Input: part model. Units: mm. Frame: model coordinates. A direction names the side the tool comes from. Give positions to 0.01 mm unless a question says otherwise; leave off trailing zeros. Loops run counter-clockwise (first coordinate to the right, second up) from the corner with the lowest first, then second, coordinate; pieces in that order, holes last. Notation, with made-up numbers: M 6,-12.5 L 58,-12.5 A31 cw 58,26.5 Z; hole C -7,38.25 d9. An arc over 180 degrees is marked long. Answer as a JSON object with one key per item and string values. Group by question number.
1) Section query D-D on z = 8. Return loops of the section in (x, y), plus the area to 3 significant figures.
2) Draft query along Y for faces 1 (the cylindrical face through (-4.769, -21.477, 14.986)), 2 (the cylindrical face through (-19.57, -0.65, 14.99)), 3 (the flat face through (9, -9, 14)), 4 (the flat face through (2.2, -2.2, 12.1)). Return one class per face: +Y half, -Y half, draft (parallel to the pull), parting line (faces both ways), or undercut.
3) Section query A-A on y = 0. Return loops of the section in (x, z).
4) First-contact query: P1, Ø2, axis at x = 6.5, z = 12.5, coming from the -Y side; P2, Ø6, axis at x = 8, y = -10, coming from the -Z side; P3, Ø2, axis at y = 4, z = 8, coming from the +X side; P4, Ø9, axis at x = 0, y = 0, coming from the +Z side. Flat tips, straight axial feed; report the tip coordinate or a pass-through.
5) Access query for faces 5 (the cylindrical face through (-1.08, -4.88, 14.08)), 6 (the flat face through (-5.2, 0.3, 16)), 7 (the cylindrical face through (-2.38, -10.74, 6.66)). Directions: +Z, -Z, +X, -X, +Y, -Y. A direction counts if a zero-diameter tool reaches every point of the face in a straight line with its end or side. Return the directions, or none.
6) Ray query, L1, parallel to Y at x = 0, z = 15.3; L2, parallel to Z at x = -6.5, y = 14; L3, parallel to Y at x = -1, z = 9.25. Return the intervals inside material, ascending.
7) Section query C-C on x = 18. Return loops of the section in (y, z).
from build123d import *

# Parameters (mm, degrees)
SKETCH1_R                                            = 11
BOSS_EXTRUDE1_DEPTH                                  = 14
SKETCH2_R                                            = 22
BOSS_EXTRUDE2_DEPTH                                  = 2
M3_CLEARANCE_HOLE1_D                                 = 3.4
CBORE_FOR_M5_HEX_SOCKET_THIN_HEAD_CAP_SC_D           = 5.5
CBORE_FOR_M5_HEX_SOCKET_THIN_HEAD_CAP_SC_CBORE_D     = 10
CBORE_FOR_M5_HEX_SOCKET_THIN_HEAD_CAP_SC_CBORE_DEPTH = 3.9
FILLET1_R                                            = 0.5


with BuildPart() as part:
    # Sketch1 → Boss-Extrude1 (new body)
    with BuildSketch(Plane.XY):
        Circle(SKETCH1_R)
    extrude(amount=BOSS_EXTRUDE1_DEPTH)

    # Sketch2 → Boss-Extrude2 (add)
    with BuildSketch(Plane.XY.offset(14)):
        Circle(SKETCH2_R)
    extrude(amount=BOSS_EXTRUDE2_DEPTH)

    # M3 Clearance Hole1 (through all)
    with Locations(Plane.XY.offset(16)):
        with Locations((-18, 0), (0, 18), (18, 0), (0, -18)):
            Hole(M3_CLEARANCE_HOLE1_D / 2)

    # CBORE for M5 Hex Socket Thin Head Cap Screw1 (through all)
    with Locations(Plane.XY.offset(16)):
        with Locations((0, 0)):
            CounterBoreHole(CBORE_FOR_M5_HEX_SOCKET_THIN_HEAD_CAP_SC_D / 2, CBORE_FOR_M5_HEX_SOCKET_THIN_HEAD_CAP_SC_CBORE_D / 2, CBORE_FOR_M5_HEX_SOCKET_THIN_HEAD_CAP_SC_CBORE_DEPTH)

    # Fillet1
    fillet1_edges = [part.edges().sort_by_distance(p)[0] for p in [
        (-11, 0, 14),
    ]]
    fillet(fillet1_edges, radius=FILLET1_R)


solid = part.part
Output:
{
 "1": {"outline": "C 0,0 d22; hole C 0,0 d5.5", "area": "356 mm^2"},
 "2": {"face 1": "parting line", "face 2": "undercut", "face 3": "draft", "face 4": "undercut"},
 "3": {"outline": "M -22,14 L -19.7,14 L -19.7,16 L -22,16 Z; M -16.3,14 L -11.5,14 A0.5 cw -11,13.5 L -11,0 L -2.75,0 L -2.75,12.1 L -5,12.1 L -5,16 L -16.3,16 Z; M 2.75,0 L 11,0 L 11,13.5 A0.5 cw 11.5,14 L 16.3,14 L 16.3,16 L 5,16 L 5,12.1 L 2.75,12.1 Z; M 19.7,14 L 22,14 L 22,16 L 19.7,16 Z"},
 "4": {"P1": "stops at y = -9.53", "P2": "stops at z = 0", "P3": "stops at x = 10.58", "P4": "stops at z = 12.1"},
 "5": {"face 5": "+Z", "face 6": "+Z, +X, -X, +Y, -Y", "face 7": "-Z"},
 "6": {"L1": "y = -22 to -19.7, -16.3 to -5, 5 to 16.3, 19.7 to 22", "L2": "z = 14 to 16", "L3": "y = -10.95 to -2.56, 2.56 to 10.95"},
 "7": {"outline": "M -12.65,14 L -1.7,14 L -1.7,16 L -12.65,16 Z; M 1.7,14 L 12.65,14 L 12.65,16 L 1.7,16 Z"}
}
